```python
from build123d import *

# Parameters (mm, degrees)
SKETCH2_R               = 17.5
BOSS_EXTRUDE1_DEPTH     = 7.5
FILLET1_R               = 3
CUT_EXTRUDE1_DEPTH      = 26.860201082
CUT_EXTRUDE1_DEPTH_BACK = 26.860201082
SKETCH4_R               = 3.448
CHAMFER1_SIZE           = 1


with BuildPart() as part:
    # Sketch2 → Boss-Extrude1 (new, symmetric)
    with BuildSketch(Plane(origin=(0, 0, 0), x_dir=(1, 0, 0), z_dir=(0, 1, 0))):
        with Locations(Location((0, 0, 0), (0, 0, 270))):
            Circle(SKETCH2_R)
    extrude(amount=BOSS_EXTRUDE1_DEPTH, both=True)

    # Fillet1
    fillet1_edges = [part.edges().sort_by_distance(p)[0] for p in [
        (0, -7.5, -17.5),
        (0, 7.5, -17.5),
    ]]
    fillet(fillet1_edges, radius=FILLET1_R)

    # Sketch4 → Cut-Extrude1 (cut, two sides: drawn at the far end of the back side and taken through both)
    with BuildSketch(Plane(origin=(0, 0, 0), x_dir=(1, 0, 0), z_dir=(0, 1, 0)).offset(-CUT_EXTRUDE1_DEPTH_BACK)):
        with Locations(Location((0, 0, 0), (0, 0, 270))):
            Circle(SKETCH4_R)
    extrude(amount=CUT_EXTRUDE1_DEPTH + CUT_EXTRUDE1_DEPTH_BACK, mode=Mode.SUBTRACT)

    # Chamfer1
    chamfer1_edges = [part.edges().sort_by_distance(p)[0] for p in [
        (0, -7.5, -3.448),
        (0, 7.5, -3.448),
    ]]
    chamfer(chamfer1_edges, length=CHAMFER1_SIZE)


solid = part.part
```
CAD build for the part. Positions are in the model's coordinates, mm. Coordinates: 2 decimals unless noted, no trailing zeros. Order: outer loops, then holes, each group sorted by start corner. A loop starts at its lowest first (then second) coordinate and runs counter-clockwise, first axis right, second up. Notation, with made-up numbers: M -17.75,-34 L 7.25,-34 A20 ccw 7.25,-16 Z; hole C 15,26 d11. An arc over 180 degrees is marked long. Answer as CSV lines item,"result".
1) Drill centre lines: L1, parallel to X at y = -0.5, z = 0; L2, parallel to Z at x = -1, y = -3.25; L3, parallel to Z at x = 2.5, y = -1.75. Where is each one in solid material? Low to high. Write a range as from..to.
Verdict:
L1,"-17.5..-3.45, 3.45..17.5"
L2,"-17.47..-3.3, 3.3..17.47"
L3,"-17.32..-2.37, 2.37..17.32"
2) Cut at B-B (x = 0). List the corners of the cut face in (y, z).
Verdict:
outline,"M -7.5,-14.5 A3 ccw -4.5,-17.5 L 4.5,-17.5 A3 ccw 7.5,-14.5 L 7.5,-4.45 L 6.5,-3.45 L -6.5,-3.45 L -7.5,-4.45 Z; M -7.5,4.45 L -6.5,3.45 L 6.5,3.45 L 7.5,4.45 L 7.5,14.5 A3 ccw 4.5,17.5 L -4.5,17.5 A3 ccw -7.5,14.5 Z"
3) Cut at D-D (y = -6). List the corners of the cut face in (x, z).
Verdict:
outline,"C 0,0 d34.2; hole C 0,0 d6.9"
4) Cut at C-C (y = -1.5). List the corners of the cut face in (x, z).
Verdict:
outline,"C 0,0 d35; hole C 0,0 d6.9"
5) Cut at A-A (z = 0). List the corners of the cut face in (x, y), then the cut area to 3 significant figures.
Verdict:
outline,"M -17.5,-4.5 A3 ccw -14.5,-7.5 L -4.45,-7.5 L -3.45,-6.5 L -3.45,6.5 L -4.45,7.5 L -14.5,7.5 A3 ccw -17.5,4.5 Z; M 3.45,-6.5 L 4.45,-7.5 L 14.5,-7.5 A3 ccw 17.5,-4.5 L 17.5,4.5 A3 ccw 14.5,7.5 L 4.45,7.5 L 3.45,6.5 Z"
area,"412 mm2"
6) Flat gauge pins, fed straight in: P1, Ø6, axis at x = -12, y = -1, coming from the +Z side; P2, Ø8, axis at y = -1, z = -11, coming from the -X side; P3, Ø6, axis at y = 0.5, z = 9, coming from the +X side. Where does each tip first touch, or does it go through?
Verdict:
P1,"z = 15.01"
P2,"x = -16.04"
P3,"x = 16.44"
7) Mould opens along X. For faces 1 (the cylindrical face through (-10.648, 0.063, -13.887)), 2 (the flat face through (3.4, -7.5, -3.4)), 3 (the cylindrical face through (1, -0.1, 3.3)) say: released by +X, released by -X, zero draft, split by the parting line, or undercut.
Verdict:
face 1,"split by the parting line"
face 2,"zero draft"
face 3,"undercut"
